Geometry check sheet. Reference: the model listing, model coordinates, mm. A direction names the side the tool comes from. Give positions to 0.01 mm unless a question says otherwise; leave off trailing zeros. Order: outer loops, then holes, each group sorted by start corner. A loop starts at its lowest first (then second) coordinate and runs counter-clockwise, first axis right, second up. Notation, with made-up numbers: M -14,66.5 L -8,66.5 A15 ccw -8,85.5 Z; hole C -18,-0.75 d5. An arc over 180 degrees is marked long. Answer as CSV lines item,"result". Start each with the question number.
Q1. Go/stop test with flat-tipped pins: pin 1 (5 mm diameter, centred on x = 3.5, y = -15.5, fed in from -Z); pin 2 (10 mm diameter, centred on y = -5.5, z = 51, fed in from +X); pin 3 (10 mm diameter, centred on y = 14.5, z = 21, fed in from +X) (3 decimals); pin 4 (4 mm diameter, centred on x = 22, y = 41.5, fed in from +Z). Record where each tip stops, or that it passes through.
Q2. Thickness scan on line 1 (X direction, y = 25, z = 14); line 2 (Y direction, x = -31, z = 35.5); line 3 (Z direction, x = 18.5, y = -32.5). Record the ranges inside material, lowest first.
Q3. Set-up check for faces 4 (the flat face through (14.82, -36.36, 35.96)), 5 (the flat face through (17.029, 40.446, 35.045)), 6 (the flat face through (-40.446, 17.029, 35.045)), 7 (the flat face through (-42, -17, 3)): record each of +Z, -Z, +X, -X, +Y, -Y from which the full face is reachable in a straight line by a thin tool's end or side.
Q4. Section check B-B, the plane y = 21.5. Record the boundary of the cut face in (x, z), then the cut area to 3 significant figures.
Q5. Mould release check, pull along X, two halves, no side actions. Record for faces 1 (the flat face through (-17, -42, 3)), 2 (the flat face through (-41.867, 1.529, 35.955)), 3 (the flat face through (40.446, -17.029, 35.045)): +X half, -X half, draft (parallel to the pull), parting line (faces both ways), or undercut.
Q6. Section check C-C, the plane x = 3. Record the boundary of the cut face in (y, z), then the cut area to 3 significant figures.
Q7. Section check A-A, the plane z = 59.5. Record the boundary of the cut face in (x, y) (3 decimals).
Autodesk Fusion 360 part; units mm, degrees
sketch "Sketch1" plane through (0, 0, 0) normal (0, 0, 1) x (1, 0, 0)
  circle A0 centre (0, 0) radius 47.5
  dimension "d1" = 95
extrude "Extrude1" add sketch "Sketch1" along normal blind 3
sketch "Sketch4" plane through (0, 0, 3) normal (0, 0, 1) x (-1, 0, 0)
  circle A0 centre (0, 0) radius 47.5
  line L0 (-47.5, 0) -> (-33.5876, -33.5876)
  line L1 (-33.5876, -33.5876) -> (0, -47.5)
  line L2 (0, -47.5) -> (33.5876, -33.5876)
  line L3 (33.5876, -33.5876) -> (47.5, 0)
  line L4 (47.5, 0) -> (33.5876, 33.5876)
  line L5 (33.5876, 33.5876) -> (0, 47.5)
  line L6 (0, 47.5) -> (-33.5876, 33.5876)
  line L7 (-33.5876, 33.5876) -> (-47.5, 0)
  dimension "d5" = 47.5
extrude "Extrude2" add sketch "Sketch4" along normal blind 65 contours L0 L1 L2 L3 L4 L5 L6 L7
sketch "Sketch5" plane through (0, 0, 68) normal (0, 0, 1) x (-1, 0, 0)
  line L0 (-33.5876, 33.5876) -> (-47.5, 0)
  line L1 (-47.5, 0) -> (-33.5876, -33.5876)
  line L2 (-33.5876, -33.5876) -> (0, -47.5)
  line L3 (0, -47.5) -> (33.5876, -33.5876)
  line L4 (33.5876, -33.5876) -> (47.5, 0)
  line L5 (47.5, 0) -> (33.5876, 33.5876)
  line L6 (33.5876, 33.5876) -> (0, 47.5)
  line L7 (0, 47.5) -> (-33.5876, 33.5876)
  line L8 (42.5, 0) -> (30.052, 30.052)
  line L9 (30.052, 30.052) -> (0, 42.5)
  line L10 (0, 42.5) -> (-30.052, 30.052)
  line L11 (-30.052, 30.052) -> (-42.5, 0)
  line L12 (-42.5, 0) -> (-30.052, -30.052)
  line L13 (-30.052, -30.052) -> (0, -42.5)
  line L14 (0, -42.5) -> (30.052, -30.052)
  line L15 (30.052, -30.052) -> (42.5, 0)
  dimension "d8" = 42.5
extrude "Extrude3" cut sketch "Sketch5" against normal blind 65 contours L8 L9 L10 L11 L12 L13 L14 L15
sketch "Sketch6" plane through (-36.276, 15.026, 0) normal (0.9239, -0.3827, 0) x (0.3827, 0.9239, 0)
  line L0 (16.264, 68) -> (-16.264, 68)
  line L1 (-16.264, 68) -> (-16.264, 3)
  line L2 (-16.264, 3) -> (16.264, 3)
  line L3 (16.264, 3) -> (16.264, 68)
  line L4 (-16.264, 68) -> (16.264, 68)
  line L5 (0, 68) -> (-11, 68)
  line L6 (0, 68) -> (11, 68)
  line L7 (11, 68) -> (13, 68)
  line L8 (13, 68) -> (13, 3)
  line L9 (13, 3) -> (11, 3)
  line L10 (-11, 68) -> (-13, 68)
  line L11 (-13, 68) -> (-13, 3)
  line L12 (-13, 3) -> (-11, 3)
  line L13 (-13, 68) -> (-11.25, 68)
  line L14 (-11.25, 68) -> (-11.25, 3)
  line L15 (-11.25, 3) -> (-13, 3)
  line L16 (-13, 3) -> (-13, 68)
  line L17 (13, 68) -> (11.25, 68)
  line L18 (11.25, 68) -> (11.25, 3)
  line L19 (11.25, 3) -> (13, 3)
  line L20 (13, 3) -> (13, 68)
  dimension "d11" = 11
  dimension "d12" = 11
  dimension "d13" = 2
  dimension "d14" = 65
  dimension "d25" = 1.75
  dimension "d26" = 65
  dimension "d27" = 1.75
  dimension "d28" = 65
extrude "Extrude4" add sketch "Sketch6" along normal blind 1.5 contours L0 L2 L4 L7 L8 L9 L17 L18 L19 L20 | L0 L2 L4 L10 L11 L12 L13 L14 L15 L16
sketch "Sketch7" plane through (-34.8902, 14.452, 0) normal (0.9239, -0.3827, 0) x (0.3827, 0.9239, 0)
  line L0 (-11.25, 68) -> (-13, 68)
  line L1 (-13, 68) -> (-13, 3)
  line L2 (-13, 3) -> (-11.25, 3)
  line L3 (-13, 68) -> (-10, 68)
  line L4 (-10, 68) -> (-10, 3)
  line L5 (-10, 3) -> (-13, 3)
  line L6 (-13, 3) -> (-13, 68)
  line L7 (-11.25, 3) -> (-11.25, 68)
  dimension "d17" = 3
  dimension "d18" = 65
extrude "Extrude5" add sketch "Sketch7" along normal blind 1
sketch "Sketch8" plane through (-34.8902, 14.452, 0) normal (0.9239, -0.3827, 0) x (0.3827, 0.9239, 0)
  line L0 (11.25, 3) -> (13, 3)
  line L1 (13, 68) -> (11.25, 68)
  line L2 (13, 68) -> (10, 68)
  line L3 (10, 68) -> (10, 3)
  line L4 (10, 3) -> (13, 3)
  line L5 (13, 3) -> (13, 68)
  line L6 (13, 3) -> (13, 68)
  line L7 (11.25, 68) -> (11.25, 3)
  dimension "d21" = 3
  dimension "d22" = 65
extrude "Extrude6" add sketch "Sketch8" along normal blind 1
Answer block:
1,pin 1,"stops at z = 0"
1,pin 2,"stops at x = 47.29"
1,pin 3,"stops at x = 43.565"
1,pin 4,"stops at z = 3"
2,line 1,"x = -37.14 to -32.14, -30.96 to -29.44, 32.14 to 37.14"
2,line 2,"y = -34.66 to -27.76, 23.66 to 23.84, 25.02 to 26.91, 27.76 to 34.66"
2,line 3,"z = 0 to 3"
3,face 4,"+Z"
3,face 5,"+Z, +X, +Y"
3,face 6,"+Z, -X, +Y"
3,face 7,"+Z, -X, -Y"
4,outline,"M -42.36,0 L 42.36,0 L 42.36,3 L 38.59,3 L 38.59,68 L 33.59,68 L 33.59,3 L -33.59,3 L -33.59,68 L -38.59,68 L -38.59,3 L -42.36,3 Z"
4,area,"904 mm2"
5,face 1,"draft"
5,face 2,"undercut"
5,face 3,"+X half"
6,outline,"M -47.41,0 L 47.41,0 L 47.41,3 L 46.26,3 L 46.26,68 L 41.26,68 L 41.26,3 L -41.26,3 L -41.26,68 L -46.26,68 L -46.26,3 L -47.41,3 Z"
6,area,"934 mm2"
7,outline,"M -47.5,0 L -33.588,-33.588 L 0,-47.5 L 33.588,-33.588 L 47.5,0 L 33.588,33.588 L 0,47.5 L -33.588,33.588 Z; hole M -42.5,0 L -30.052,-30.052 L 0,-42.5 L 30.052,-30.052 L 42.5,0 L 30.052,30.052 L 0,42.5 L -30.052,30.052 L -31.301,27.036 L -28.991,26.08 L -30.139,23.308 L -31.063,23.691 L -30.585,24.846 L -31.971,25.42 L -40.581,4.632 L -39.195,4.058 L -38.717,5.213 L -37.793,4.831 L -38.941,2.059 L -41.251,3.016 Z"
